Input: part model. Units: mm. Frame: model coordinates. Give positions to 0.01 mm unless a question says otherwise; leave off trailing zeros. Loops run counter-clockwise (first coordinate to the right, second up) from the corner with the lowest first, then second, coordinate; pieces in that order, holes last.
from build123d import *

# Parameters (mm, degrees)
SKETCH_1_R          = 36.5
SKETCH_1_R_2        = 6.5
EXTRUDE_1_DEPTH     = 4
SKETCH_2_R          = 1.65
CUT_EXTRUDE_1_DEPTH = 6


with BuildPart() as part:
    # 草图1 → 凸台-拉伸1 (new body)
    with BuildSketch(Plane(origin=(0, 0, 0), x_dir=(0, 0, -1), z_dir=(1, 0, 0))):
        Circle(SKETCH_1_R)
        Circle(SKETCH_1_R_2, mode=Mode.SUBTRACT)
    extrude(amount=EXTRUDE_1_DEPTH)

    # 草图2 → 切除-拉伸1 (cut)
    with BuildSketch(Plane(origin=(4, 0, 0), x_dir=(0, 0, -1), z_dir=(1, 0, 0))):
        with Locations((32.9, 0)):
            Circle(SKETCH_2_R)
        with Locations((23.263813101, -23.263813101)):
            Circle(SKETCH_2_R)
        with Locations((0, -32.9)):
            Circle(SKETCH_2_R)
        with Locations((-23.263813101, -23.263813101)):
            Circle(SKETCH_2_R)
        with Locations((-32.9, 0)):
            Circle(SKETCH_2_R)
        with Locations((-23.263813101, 23.263813101)):
            Circle(SKETCH_2_R)
        with Locations((0, 32.9)):
            Circle(SKETCH_2_R)
        with Locations((23.263813101, 23.263813101)):
            Circle(SKETCH_2_R)
    extrude(amount=-CUT_EXTRUDE_1_DEPTH, mode=Mode.SUBTRACT)


solid = part.part
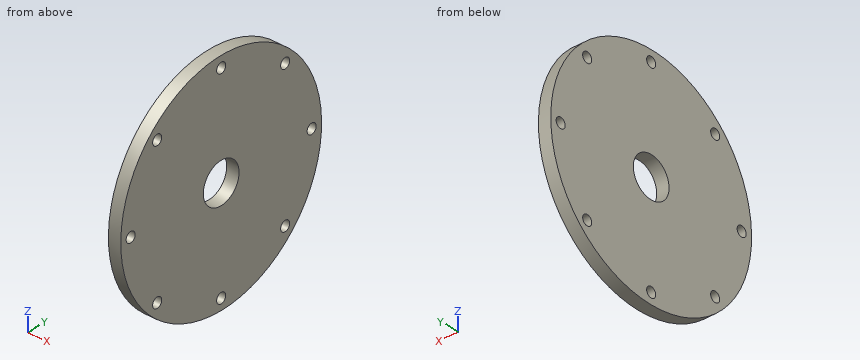
(1) Cut plane B-B (z = -22.5). Return the cut outline in (x, y), and give its area (3 significant figures).
Values follow:
outline: (0, -28.74) - (4, -28.74) - (4, -24.73) - (0, -24.73) - close; (0, -21.8) - (4, -21.8) - (4, 21.8) - (0, 21.8) - close; (0, 24.73) - (4, 24.73) - (4, 28.74) - (0, 28.74) - close
area: 207 mm2
(2) Pin query (flat end, axial travel): pin 1 Ø1.5 at (x, z) = (2, -8) entering from +Y; pin 2 Ø2 at (y, z) = (23.26, 23.26) entering from -X; pin 3 Ø1.5 at (x, y) = (3.5, -19.5) entering from -Z; pin 4 Ø4 at (y, z) = (-32.9, 0) entering from -X. Return the tip coordinate at first contact, or that it passes through.
Values follow:
pin 1: stops at y = 35.77
pin 2: passes through
pin 3: stops at z = -31.32
pin 4: stops at x = 0
(3) Ray query, probe 1 along Y at (x, z) = (0.7, 0); probe 2 along Z at (x, y) = (2.65, 1); probe 3 along Z at (x, y) = (3.1, -23). Return the intervals inside material, ascending.
Values follow:
probe 1: y = -36.5 to -34.55, -31.25 to -6.5, 6.5 to 31.25, 34.55 to 36.5
probe 2: z = -36.49 to -34.21, -31.59 to -6.42, 6.42 to 31.59, 34.21 to 36.49
probe 3: z = -28.34 to -24.89, -21.64 to 21.64, 24.89 to 28.34
(4) Cut plane A-A (y = 0). Return the cut outline in (x, z).
Values follow:
outline: (0, -36.5) - (4, -36.5) - (4, -34.55) - (0, -34.55) - close; (0, -31.25) - (4, -31.25) - (4, -6.5) - (0, -6.5) - close; (0, 6.5) - (4, 6.5) - (4, 31.25) - (0, 31.25) - close; (0, 34.55) - (4, 34.55) - (4, 36.5) - (0, 36.5) - close
(5) Cut plane C-C (y = -32.9). Return the cut outline in (x, z).
Values follow:
outline: (0, -15.81) - (4, -15.81) - (4, -1.65) - (0, -1.65) - close; (0, 1.65) - (4, 1.65) - (4, 15.81) - (0, 15.81) - close
